The listing builds one solid part. Answer for the finished solid, in the listing's coordinates (mm). Face numbers are marked on the shaded views. A direction names the side the tool comes from. Give positions to 0.01 mm unless a question says otherwise; leave off trailing zeros. Write each loop counter-clockwise with the first axis right and the second up, starting at its lowest first coordinate (ties: lowest second). Pieces come first, ordered by that corner, then holes.
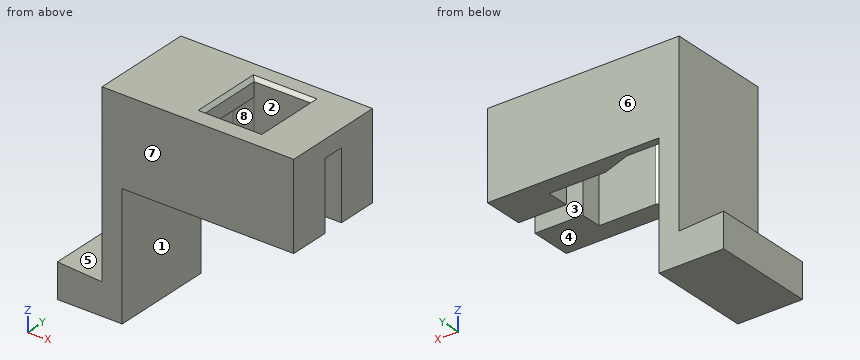
```python
from build123d import *

# Parameters (mm, degrees)
F0_W     = 27.94
F0_H     = 15
F0_W_2   = 8.25
F0_H_2   = 9.5
F1_DEPTH = 2.54
F2_W     = 1.7651973286
F2_H     = 4.826
F2_W_2   = 1.3194764033
F3_DEPTH = 10
F4_W     = 2.94
F4_H     = 15
F5_DEPTH = 18
F6_W     = 15
F6_H     = 5
F7_DEPTH = 6.5
F9_DEPTH = 25.4
F10_SIZE = 0.508


# Not quite as in the source:
# - a feature names something its author has since deleted; it is built from what else it names


with BuildPart() as f1:
    # F0 (on Top) → F1 (new body)
    with BuildSketch(Plane.XY):
        with Locations((2.7402517554, 4.2405291848)):
            Rectangle(F0_W, F0_H)
        with Locations((5.5952517554, 4.3655291848)):
            Rectangle(F0_W_2, F0_H_2, mode=Mode.SUBTRACT)
    extrude(amount=F1_DEPTH)

    # F2 (on face) → F3 (join)
    with BuildSketch(Plane(origin=(0, 0, 0), x_dir=(1, 0, 0), z_dir=(0, 0, -1))):
        Polygon((-11.2297482446, -11.7405291848), (16.7102517554, -11.7405291848), (16.7102517554, -10.6549952576), (14.9450544268, -10.6549952576), (13.6255780235, -10.6549952576), (-2.7816970833, -10.6549952576), (-8.2897482446, -10.6549952576), (-11.2297482446, -10.6549952576), align=None)
        with Locations((15.8276530911, -8.2419952576)):
            Rectangle(F2_W, F2_H)
        with Locations((15.8276530911, -0.3159952576)):
            Rectangle(F2_W, F2_H)
        Polygon((-2.7816970833, -10.6549952576), (13.6255780235, -10.6549952576), (13.6255780235, -5.8289952576), (9.7202517554, -5.8289952576), (9.7202517554, -9.1155291848), (1.4702517554, -9.1155291848), align=None)
        Polygon((-8.2897482446, 3.2594708152), (-8.2897482446, 2.0970047424), (-2.7816970833, 2.0970047424), (13.6255780235, 2.0970047424), (14.9450544268, 2.0970047424), (16.7102517554, 2.0970047424), (16.7102517554, 3.2594708152), align=None)
        Polygon((13.6255780235, 2.0970047424), (-2.7816970833, 2.0970047424), (1.4702517554, 0.3844708152), (9.7202517554, 0.3844708152), (9.7202517554, -2.7289952576), (13.6255780235, -2.7289952576), align=None)
        with Locations((14.2853162251, -8.2419952576)):
            Rectangle(F2_W_2, F2_H)
        with Locations((14.2853162251, -0.3159952576)):
            Rectangle(F2_W_2, F2_H)
        Polygon((-11.2297482446, 3.2594708152), (-11.2297482446, -10.6549952576), (-8.2897482446, -10.6549952576), (-8.2897482446, 2.0970047424), (-8.2897482446, 3.2594708152), align=None)
    extrude(amount=F3_DEPTH)

    # F4 (on face) → F5 (join)
    with BuildSketch(Plane(origin=(0, 0, -10), x_dir=(1, 0, 0), z_dir=(0, 0, -1))):
        with Locations((-9.7597482446, -4.2405291848)):
            Rectangle(F4_W, F4_H)
    extrude(amount=F5_DEPTH)

    # F6 (on face) → F7 (join)
    with BuildSketch(Plane(origin=(-11.2297482446, 0, 0), x_dir=(0, -1, 0), z_dir=(-1, 0, 0))):
        with Locations((-4.2405291848, -25.5)):
            Rectangle(F6_W, F6_H)
    extrude(amount=F7_DEPTH)

    # F8 (on face) → F9 (cut)
    with BuildSketch(Plane.XZ.offset(3.2594708152)):
        Polygon((-11.2297482446, -23), (-17.7297482446, -23), (-11.2297482446, -23.4054420143), align=None)
    extrude(amount=-F9_DEPTH, mode=Mode.SUBTRACT)

    # F10
    f10_edges = [f1.edges().sort_by_distance(p)[0] for p in [
        (1.470252, 4.365529, 2.54),
        (5.595252, 9.115529, 2.54),
        (9.720252, 4.365529, 2.54),
        (5.595252, -0.384471, 2.54),
    ]]
    chamfer(f10_edges, length=F10_SIZE)


solid = f1.part
```
Item 1: A cutting plane is placed at A-A, the plane y = 2. Give the vertices of the cut face in (x, z).
Conclusion:
outline: (-17.73, -28) - (-8.29, -28) - (-8.29, 0) - (1.47, 0) - (1.47, 2.03) - (0.96, 2.54) - (-11.23, 2.54) - (-11.23, -23.41) - (-17.73, -23) - close; (9.72, -10) - (16.71, -10) - (16.71, 2.54) - (10.23, 2.54) - (9.72, 2.03) - close
Item 2: A cutting plane is placed at D-D, the plane z = -7. Give the vertices of the cut face in (x, y) (3 decimals).
Conclusion:
outline: (-11.23, -3.259) - (16.71, -3.259) - (16.71, 2.729) - (9.72, 2.729) - (9.72, -0.384) - (1.47, -0.384) - (-2.782, -2.097) - (-8.29, -2.097) - (-8.29, 10.655) - (-2.782, 10.655) - (1.47, 9.116) - (9.72, 9.116) - (9.72, 5.829) - (16.71, 5.829) - (16.71, 11.741) - (-11.23, 11.741) - close
Item 3: A cutting plane is placed at B-B, the plane x = 6. Give the vertices of the cut face in (y, z).
Conclusion:
outline: (-3.26, -10) - (-0.38, -10) - (-0.38, 2.03) - (-0.89, 2.54) - (-3.26, 2.54) - close; (9.12, -10) - (11.74, -10) - (11.74, 2.54) - (9.62, 2.54) - (9.12, 2.03) - close
Item 4: Consider probe 1 along Y at (x, z) = (7, -9.5); probe 2 along X at (y, z) = (6.5, -6); probe 3 along Y at (x, z) = (-4.5, -8.5) (3 decimals). Determine where each line is inside the solid, lowest interval first.
Conclusion:
probe 1: y = -3.26 to -0.38, 9.12 to 11.74
probe 2: x = -11.23 to -8.29, 9.72 to 16.71
probe 3: y = -3.259 to -2.097, 10.655 to 11.741
Item 5: Each of these flat-tipped pins is pushed along its axis until it touches: P1, Ø5, axis at x = -1.5, y = 7, coming from the -Z side; P2, Ø3, axis at x = 8, y = 0, coming from the -Z side; P3, Ø2, axis at y = 0, z = -11.5, coming from the +X side. Where does it stop, or does it pass through?
Conclusion:
P1: stops at z = 0
P2: stops at z = -10
P3: stops at x = -8.29
Item 6: A cutting plane is placed at C-C, the plane x = -4. Give the vertices of the cut face in (y, z) (3 decimals), plus the area to 3 significant figures.
Conclusion:
outline: (-3.259, -10) - (-2.097, -10) - (-2.097, 0) - (10.655, 0) - (10.655, -10) - (11.741, -10) - (11.741, 2.54) - (-3.259, 2.54) - close
area: 60.6 mm2
Item 7: Which of the six approach directions +Z, -Z, +X, -X, +Y, -Y give full straight-line access (tool end or side, diameter ignored) to the marked faces 1, 2, 3 and 4?
Conclusion:
face 1: -Z
face 2: +Z, -Z
face 3: -Z, +X
face 4: -Z, +X, +Y, -Y
Item 8: Determine the mould class of the marked faces 5, 6, 7 and 8 for opening direction Y: pulls with the +Y half, pulls with the -Y half, needs draft (parallel to the pull), parting line crosses it, or undercut.
Conclusion:
face 5: needs draft
face 6: pulls with the +Y half
face 7: pulls with the -Y half
face 8: undercut
